from build123d import *

# Parameters (mm, degrees)
F0_R     = 75
F0_R_2   = 1.5
F0_R_3   = 30
F1_DEPTH = 18
F2_R     = 4.25
F3_DEPTH = 5


with BuildPart() as f1:
    # F0 (on Top) → F1 (new body)
    with BuildSketch(Plane.XY):
        Circle(F0_R)
        with Locations((-54.126588, -31.25)):
            Circle(F0_R_2, mode=Mode.SUBTRACT)
        with Locations((54.126588, -31.25)):
            Circle(F0_R_2, mode=Mode.SUBTRACT)
        Circle(F0_R_3, mode=Mode.SUBTRACT)
        with Locations((0, 62.5)):
            Circle(F0_R_2, mode=Mode.SUBTRACT)
    extrude(amount=F1_DEPTH)

    # F2 (on face) → F3 (cut)
    with BuildSketch(Plane.XY.offset(18)):
        with Locations((-54.126588, -31.25)):
            Circle(F2_R)
        with Locations((54.126588, -31.25)):
            Circle(F2_R)
        with Locations((0, 62.5)):
            Circle(F2_R)
    extrude(amount=-F3_DEPTH, mode=Mode.SUBTRACT)


solid = f1.part
Design review of the part built by this model. Coordinates are the model's own, in mm. A direction names the side the tool comes from. Give positions to 0.01 mm unless a question says otherwise; leave off trailing zeros. Write each loop counter-clockwise with the first axis right and the second up, starting at its lowest first coordinate (ties: lowest second). Pieces come first, ordered by that corner, then holes. Notation, with made-up numbers: M 6.25,-26.5 L 34.25,-26.5 A22 ccw 34.25,-16.5 Z; hole C 69,-6.75 d11. An arc over 180 degrees is marked long. Answer as a JSON object with one key per item and string values. Group by question number.
1) Tool access review of faces 4 (the face through (2, 63, 13)), 5 (the face through (32, 1, 0)): name each direction out of +Z, -Z, +X, -X, +Y, -Y from which nothing blocks a thin tool from reaching the whole face with its end or side.
2) Mouldability with a two-part tool opening along Y and no side actions: class faces 1 (the face through (32, 1, 18)), 2 (the face through (-52, -31, 13)), 3 (the face through (-9.764, 74.362, 8.874)) as released by +Y, released by -Y, zero draft, split by the parting line, or undercut.
3) We need section A-A (y = 0). Give the boundary of the cut face in (x, z), and give its area (3 significant figures).
4) For line 1 along Y through (x, z) = (0, 5.75); line 2 along X through (y, z) = (-31.25, 10); line 3 along X through (y, z) = (4.5, 3.75), list the stretches that pass through material, from the lowest coordinate up.
5) We need section D-D (y = -37.5). Give the boundary of the cut face in (x, z), and give its area (3 significant figures).
6) Clearance check with flat-ended pins moving along their axes: pin 1 Ø5 at (x, z) = (-49.5, 4) entering from +Y; pin 2 Ø1.8 at (x, y) = (0, 62.5) entering from +Z; pin 3 Ø2 at (y, z) = (10.5, 14.5) entering from +X; pin 4 Ø2 at (y, z) = (40, 7) entering from -X. State where each tip first meets the part, or that it passes through.
7) We need section C-C (x = -11). Give the boundary of the cut face in (y, z), and give its area (3 significant figures).
8) We need section B-B (z = 7). Give the boundary of the cut face in (x, y), and give its area (3 significant figures).
Answer key:
{
 "1": {"face 4": "+Z", "face 5": "-Z, +X, -X, +Y, -Y"},
 "2": {"face 1": "zero draft", "face 2": "undercut", "face 3": "split by the parting line"},
 "3": {"outline": "M -75,0 L -30,0 L -30,18 L -75,18 Z; M 30,0 L 75,0 L 75,18 L 30,18 Z", "area": "1,620 mm²"},
 "4": {"line 1": "y = -75 to -30, 30 to 61, 64 to 75", "line 2": "x = -68.18 to -55.63, -52.63 to 52.63, 55.63 to 68.18", "line 3": "x = -74.86 to -29.66, 29.66 to 74.86"},
 "5": {"outline": "M -64.95,0 L 64.95,0 L 64.95,18 L -64.95,18 Z", "area": "2,340 mm²"},
 "6": {"pin 1": "stops at y = 58.45", "pin 2": "passes through", "pin 3": "stops at x = 74.4", "pin 4": "stops at x = -64.06"},
 "7": {"outline": "M -74.19,0 L -27.91,0 L -27.91,18 L -74.19,18 Z; M 27.91,0 L 74.19,0 L 74.19,18 L 27.91,18 Z", "area": "1,670 mm²"},
 "8": {"outline": "C 0,0 d150; hole C -54.13,-31.25 d3; hole C 0,0 d60; hole C 0,62.5 d3; hole C 54.13,-31.25 d3", "area": "14,800 mm²"}
}
